CAD build for the part. Positions are in the model's coordinates, mm. A direction names the side the tool comes from. Give positions to 0.01 mm unless a question says otherwise; leave off trailing zeros. Loops run counter-clockwise (first coordinate to the right, second up) from the corner with the lowest first, then second, coordinate; pieces in that order, holes last.
Item 1: Saw through at B-B on y = -5. Give the cut face in (x, z).
Item 2: Drop flat-ended pins along their axis: P1, Ø1, axis at x = -4.5, z = 7, coming from the +Y side; P2, Ø1.5, axis at y = -4.5, z = 8, coming from the -X side; P3, Ø4, axis at y = -5, z = -7.5, coming from the -X side; P4, Ø4, axis at y = -5.5, z = -8.5, coming from the -X side. Give the stop position or say it passes through.
Item 3: Saw through at D-D on y = -3. Give the cut face in (x, z), plus the area to 3 significant figures.
Item 4: Probe probe 1 along Y at (x, z) = (-5.7, -7.5); probe 2 along Y at (x, z) = (-2.5, -7.5); probe 3 along Z at (x, y) = (-5.35, -5). List the from-to ranges inside material, lowest first.
Item 5: Saw through at A-A on z = -7.5. Give the cut face in (x, y).
Item 6: Mould opens along Z. For faces 1 (the flat face through (-4, -5, 11)), 2 (the flat face through (-3, -5, -11)), 3 (the flat face through (-6.5, -10, -0.2)), 4 (the cylindrical face through (-3.03, -6.04, 7.36)) say: released by +Z, released by -Z, zero draft, split by the parting line, or undercut.
Item 7: Saw through at C-C on x = -3.5. Give the cut face in (y, z).
Item 8: Which spindle directions (+Z, -Z, +X, -X, +Y, -Y) get a long thin tool onto all of the face, cutting with end or side? Do faces 5 (the flat face through (-6, -5, 10)), 6 (the flat face through (-1, -5, -9)), 7 (the flat face through (-6, -5, -10)), 8 (the cylindrical face through (-5.499, -5.297, -5.775)). Say none if no direction does.
from build123d import *

# Parameters (mm, degrees)
BOSS_EXTRUDE1_DEPTH     = 10
CUT_EXTRUDE1_DEPTH      = 18.12454379
CUT_EXTRUDE1_DEPTH_BACK = 18.12454379
SKETCH2_R               = 1.05
CUT_EXTRUDE2_DEPTH      = 1
CUT_EXTRUDE2_DEPTH_BACK = 10
CUT_EXTRUDE2_START      = -6
SKETCH2_3_R             = 1.75
SKETCH2_3_R_2           = 1.05


with BuildPart() as part:
    # Sketch1 → Boss-Extrude1 (new body)
    with BuildSketch(Plane(origin=(0, 0, 0), x_dir=(1, 0, 0), z_dir=(0, 1, 0))):
        with BuildLine():
            Line((-6, -2.1e-08), (-6, 6.020797289))
            ThreePointArc((-6, 6.020797289), (-8.5, 0), (-6, -6.020797289))
            Line((-6, -6.020797289), (-6, -2.1e-08))
        make_face()
        with BuildLine():
            ThreePointArc((-1, 8.440971508), (-3.703283788, 7.65086199), (-6, 6.020797289))
            Line((-6, 6.020797289), (-6, -2.1e-08))
            ThreePointArc((-6, -2.1e-08), (-4.582575702, 3.872983338), (-1, 5.916079783))
            Line((-1, 5.916079783), (-1, 8.440971508))
        make_face()
        with BuildLine():
            ThreePointArc((-1, -5.916079783), (-4.582575688, -3.872983354), (-6, -2.1e-08))
            Line((-6, -2.1e-08), (-6, -6.020797289))
            ThreePointArc((-6, -6.020797289), (-3.703283788, -7.65086199), (-1, -8.440971508))
            Line((-1, -8.440971508), (-1, -5.916079783))
        make_face()
        with BuildLine():
            ThreePointArc((-1, -8.440971508), (-3.703283788, -7.65086199), (-6, -6.020797289))
            Line((-6, -6.020797289), (-6, -11))
            Line((-6, -11), (-1, -11))
            Line((-1, -11), (-1, -8.440971508))
        make_face()
        with BuildLine():
            Line((-1, 11), (-6, 11))
            Line((-6, 11), (-6, 6.020797289))
            ThreePointArc((-6, 6.020797289), (-3.703283788, 7.65086199), (-1, 8.440971508))
            Line((-1, 8.440971508), (-1, 11))
        make_face()
    extrude(amount=-BOSS_EXTRUDE1_DEPTH)

    # Sketch2 → Cut-Extrude1 (cut, two sides: drawn at the far end of the back side and taken through both)
    with BuildSketch(Plane(origin=(0, 0, 0), x_dir=(0, 0, -1), z_dir=(1, 0, 0)).offset(-CUT_EXTRUDE1_DEPTH_BACK)):
        with Locations(Location((-7.5, -5, 0), (0, 0, 180))):
            Circle(SKETCH2_R)
        with Locations(Location((7.5, -5, 0), (0, 0, 180))):
            Circle(SKETCH2_R)
    extrude(amount=CUT_EXTRUDE1_DEPTH + CUT_EXTRUDE1_DEPTH_BACK, mode=Mode.SUBTRACT)

    # Sketch2<3> → Cut-Extrude2 (cut, two sides: drawn at the far end of the back side and taken through both)
    # profile 1 of 2: a face of its own
    with BuildSketch(Plane(origin=(0, 0, 0), x_dir=(0, 0, -1), z_dir=(1, 0, 0)).offset(CUT_EXTRUDE2_START - CUT_EXTRUDE2_DEPTH_BACK)):
        with Locations(Location((-7.5, -5, 0), (0, 0, 327.699663161))):
            Circle(SKETCH2_3_R)
        with Locations(Location((-7.5, -5, 0), (0, 0, 180))):
            Circle(SKETCH2_3_R_2, mode=Mode.SUBTRACT)
    # profile 2 of 2: a face of its own
    with BuildSketch(Plane(origin=(0, 0, 0), x_dir=(0, 0, -1), z_dir=(1, 0, 0)).offset(CUT_EXTRUDE2_START - CUT_EXTRUDE2_DEPTH_BACK)):
        with Locations(Location((7.5, -5, 0), (0, 0, 212.300336839))):
            Circle(SKETCH2_3_R)
        with Locations(Location((7.5, -5, 0), (0, 0, 180))):
            Circle(SKETCH2_3_R_2, mode=Mode.SUBTRACT)
    extrude(amount=CUT_EXTRUDE2_DEPTH + CUT_EXTRUDE2_DEPTH_BACK, mode=Mode.SUBTRACT)


solid = part.part
Results below:
1. outline: (-6.26, -5.75) - (-5, -5.75) - (-5, -6.45) - (-1, -6.45) - (-1, -5.92) arc R6 cw to (-1, 5.92) - (-1, 6.45) - (-5, 6.45) - (-5, 5.75) - (-6.26, 5.75) arc R8.5 ccw to start; (-6, -11) - (-1, -11) - (-1, -8.55) - (-5, -8.55) - (-5, -9.25) - (-6, -9.25) - close; (-6, 9.25) - (-5, 9.25) - (-5, 8.55) - (-1, 8.55) - (-1, 11) - (-6, 11) - close
2. P1: stops at y = 0
2. P2: stops at x = -5
2. P3: stops at x = -6.48
2. P4: stops at x = -6
3. outline: (-6, -11) - (-1, -11) - (-1, -5.92) arc R6 cw to (-1, 5.92) - (-1, 11) - (-6, 11) - (-6, 6.02) arc R8.5 ccw to (-6, -6.02) - close
3. area: 86.1 mm2
4. probe 1: y = -10 to -6.75, -3.25 to 0
4. probe 2: y = -10 to -6.05, -3.95 to 0
4. probe 3: z = -11 to -9.25, -5.75 to -2.72, 2.72 to 5.75, 9.25 to 11
5. outline: (-6, -10) - (-1, -10) - (-1, -6.05) - (-5, -6.05) - (-5, -6.75) - (-6, -6.75) - close; (-6, -3.25) - (-5, -3.25) - (-5, -3.95) - (-1, -3.95) - (-1, 0) - (-6, 0) - close
6. face 1: released by +Z
6. face 2: released by -Z
6. face 3: zero draft
6. face 4: undercut
7. outline: (-10, -11) - (0, -11) - (0, -4.87) - (-10, -4.87) - close; (-10, 4.87) - (0, 4.87) - (0, 11) - (-10, 11) - close; hole circle Ø2.1 at (-5, -7.5); hole circle Ø2.1 at (-5, 7.5)
8. face 5: +Z, -X, +Y, -Y
8. face 6: +Z, -Z, +X, +Y, -Y
8. face 7: -Z, -X, +Y, -Y
8. face 8: -X
